```python
from build123d import *

# Parameters (mm, degrees)
SKETCH_1_W          = 40
SKETCH_1_H          = 39
SKETCH_1_R          = 2
EXTRUDE_2_DEPTH     = 20
SKETCH_4_R          = 2
CUT_EXTRUDE_1_DEPTH = 20
SKETCH_5_R          = 4
EXTRUDE_3_DEPTH     = 1
SKETCH_6_R          = 3
EXTRUDE_4_DEPTH     = 0.5
SKETCH_7_R          = 1.5
EXTRUDE_5_DEPTH     = 4.5
FILLET_2_R          = 3
FILLET_3_R          = 3
FILLET_4_R          = 1
FILLET_5_R          = 1
FILLET_6_R          = 1
FILLET_8_R          = 1


with BuildPart() as part:
    # 草图1 → 凸台-拉伸2 (new body)
    with BuildSketch(Plane.XY):
        Rectangle(SKETCH_1_W, SKETCH_1_H)
        with BuildLine():
            Line((-20, 7.5), (-20, 11.5))
            Line((-20, 11.5), (-24, 11.5))
            ThreePointArc((-24, 11.5), (-22.585786438, 10.914213562), (-22, 9.5))
            ThreePointArc((-22, 9.5), (-22.585786438, 8.085786438), (-24, 7.5))
            Line((-24, 7.5), (-20, 7.5))
        make_face()
        with BuildLine():
            ThreePointArc((-24, 7.5), (-26, 9.5), (-24, 11.5))
            Line((-24, 11.5), (-27, 11.5))
            Line((-27, 11.5), (-27, 7.5))
            Line((-27, 7.5), (-24, 7.5))
        make_face()
        with Locations((-24, 9.5)):
            Circle(SKETCH_1_R)
        Polygon((27, 11.5), (20, 11.5), (20, 7.5), (24, 7.5), (27, 7.5), align=None)
    extrude(amount=EXTRUDE_2_DEPTH)

    # 草图4 → 切除-拉伸1 (cut)
    with BuildSketch(Plane(origin=(0, 19.5, 0), x_dir=(1, 0, 0), z_dir=(0, 1, 0))):
        with Locations((-24, -15)):
            Circle(SKETCH_4_R)
        with Locations((24, -15)):
            Circle(SKETCH_4_R)
        with Locations((-24, -5)):
            Circle(SKETCH_4_R)
        with Locations((24, -5)):
            Circle(SKETCH_4_R)
    extrude(amount=-CUT_EXTRUDE_1_DEPTH, mode=Mode.SUBTRACT)

    # 草图5 → 凸台-拉伸3 (add)
    with BuildSketch(Plane(origin=(0, 19.5, 0), x_dir=(1, 0, 0), z_dir=(0, 1, 0))):
        with Locations((-10, -10)):
            Circle(SKETCH_5_R)
    extrude(amount=EXTRUDE_3_DEPTH)

    # 草图6 → 凸台-拉伸4 (add)
    with BuildSketch(Plane(origin=(0, 20.5, 0), x_dir=(1, 0, 0), z_dir=(0, 1, 0))):
        with Locations((-10, -10)):
            Circle(SKETCH_6_R)
    extrude(amount=EXTRUDE_4_DEPTH)

    # 草图7 → 凸台-拉伸5 (add)
    with BuildSketch(Plane(origin=(0, 21, 0), x_dir=(1, 0, 0), z_dir=(0, 1, 0))):
        with Locations((-10, -10)):
            Circle(SKETCH_7_R)
    extrude(amount=EXTRUDE_5_DEPTH)

    # 圆角2
    fillet_2_edges = [part.edges().sort_by_distance(p)[0] for p in [
        (-20, 15.5, 20),
    ]]
    fillet(fillet_2_edges, radius=FILLET_2_R)

    # 圆角3
    fillet_3_edges = [part.edges().sort_by_distance(p)[0] for p in [
        (-20, 15.5, 0),
        (20, 15.5, 0),
        (20, 15.5, 20),
    ]]
    fillet(fillet_3_edges, radius=FILLET_3_R)

    # 圆角4
    fillet_4_edges = [part.edges().sort_by_distance(p)[0] for p in [
        (20, -6, 0),
        (0, -19.5, 0),
        (-20, -6, 0),
        (20, -19.5, 10),
        (-20, -19.5, 10),
        (-20, -6, 20),
        (0, -19.5, 20),
        (20, -6, 20),
    ]]
    fillet(fillet_4_edges, radius=FILLET_4_R)

    # 圆角5
    fillet_5_edges = [part.edges().sort_by_distance(p)[0] for p in [
        (-27, 9.5, 0),
        (-27, 9.5, 20),
    ]]
    fillet(fillet_5_edges, radius=FILLET_5_R)

    # 圆角6
    fillet_6_edges = [part.edges().sort_by_distance(p)[0] for p in [
        (19.121320344, 19.5, 0.878679656),
        (19.121320344, 19.5, 19.121320344),
        (0, 19.5, 20),
        (-20, 19.5, 10),
        (-19.121320344, 19.5, 19.121320344),
        (20, 19.5, 10),
        (0, 19.5, 0),
        (-19.121320344, 19.5, 0.878679656),
    ]]
    fillet(fillet_6_edges, radius=FILLET_6_R)

    # 圆角8
    fillet_8_edges = [part.edges().sort_by_distance(p)[0] for p in [
        (27, 9.5, 0),
        (27, 9.5, 20),
    ]]
    fillet(fillet_8_edges, radius=FILLET_8_R)


solid = part.part
```
Work out the finished part from the listing and answer in its coordinate system (mm). A direction names the side the tool comes from. Round coordinates to 2 decimals unless told otherwise and drop trailing zeros. Loops run counter-clockwise (first coordinate to the right, second up) from the corner with the lowest first, then second, coordinate; pieces in that order, holes last. Notation, with made-up numbers: (47, 56) -> (53, 56) arc R21 cw to (53, 86) -> close; hole circle Ø6 at (15.25, 74.5). An arc over 180 degrees is marked (long way). Write each question's results on one line, items separated by ' | '. Start each with the question number.
1. Section C-C (y = 0) is taken. Determine the outline of the cut face in (x, z).
2. For a pull along Z with two mould halves and no side action, classify faces 5 (the face through (0, -19.5, 10)), 6 (the face through (-25.474, 9.528, 13.648)), 7 (the face through (0, 0, 0)) as +Z half, -Z half, draft (parallel to the pull), parting line (faces both ways), or undercut.
3. Find the intervals of material crossed by probe 1 along X at (y, z) = (9.15, 15); probe 2 along Z at (x, y) = (24, 8.85); probe 3 along X at (y, z) = (8.5, 14), in increasing order. Write a range as from..to.
4. Given pin 1 Ø8 at (x, z) = (-23, 11) entering from +Y; pin 2 Ø2 at (y, z) = (13.5, 7.5) entering from +X; pin 3 Ø5 at (y, z) = (-12.5, 7.5) entering from -X; pin 4 Ø3.5 at (x, z) = (24, 5) entering from +Y, each flat-ended and moving along its own axis, determine where each tip first touches the part or whether it passes through.
5. A tool of negligible diameter and unlimited length cuts with its end or side. For faces 1 (the face through (-20, -6, 10)), 2 (the face through (20, 15, 10)), 3 (the face through (-8.7, 21, 11.3)), 4 (the face through (20, -6, 10)), from which of +Z, -Z, +X, -X, +Y, -Y can it reach the whole face along a straight path? Write none if from no direction.
6. Section A-A (x = 24) is taken. Determine the outline of the cut face in (y, z), plus the area to 3 significant figures.
7. Section B-B (z = 5) is taken. Determine the outline of the cut face in (x, y).
8. Section D-D (x = -10) is taken. Determine the outline of the cut face in (y, z).
Evaluation:
1) outline: (-20, 1) arc R1 ccw to (-19, 0) -> (19, 0) arc R1 ccw to (20, 1) -> (20, 19) arc R1 ccw to (19, 20) -> (-19, 20) arc R1 ccw to (-20, 19) -> close
2) face 5: draft | face 6: undercut | face 7: -Z half
3) probe 1: x = -27..-26, -22..22, 26..27 | probe 2: z = 0..3, 7..13, 17..20 | probe 3: x = -27..-25.73, -22.27..22.27, 25.73..27
4) pin 1: stops at y = 19.5 | pin 2: stops at x = 20 | pin 3: stops at x = -20 | pin 4: passes through
5) face 1: +Z, -Z, -X, -Y | face 2: +Z, -Z, +X, +Y | face 3: +Y | face 4: +Z, -Z, +X, -Y
6) outline: (7.5, 0) -> (11.5, 0) -> (11.5, 3) -> (7.5, 3) -> close; (7.5, 7) -> (11.5, 7) -> (11.5, 13) -> (7.5, 13) -> close; (7.5, 17) -> (11.5, 17) -> (11.5, 20) -> (7.5, 20) -> close | area: 48.0 mm2
7) outline: (-27, 7.5) -> (-26, 7.5) -> (-26, 11.5) -> (-27, 11.5) -> close; (-22, 7.5) -> (-20, 7.5) -> (-20, -18.5) arc R1 ccw to (-19, -19.5) -> (19, -19.5) arc R1 ccw to (20, -18.5) -> (20, 7.5) -> (22, 7.5) -> (22, 11.5) -> (20, 11.5) -> (20, 18.5) arc R1 ccw to (19, 19.5) -> (-19, 19.5) arc R1 ccw to (-20, 18.5) -> (-20, 11.5) -> (-22, 11.5) -> close; (26, 7.5) -> (27, 7.5) -> (27, 11.5) -> (26, 11.5) -> close
8) outline: (-19.5, 1) arc R1 ccw to (-18.5, 0) -> (18.5, 0) arc R1 ccw to (19.5, 1) -> (19.5, 6) -> (20.5, 6) -> (20.5, 7) -> (21, 7) -> (21, 8.5) -> (25.5, 8.5) -> (25.5, 11.5) -> (21, 11.5) -> (21, 13) -> (20.5, 13) -> (20.5, 14) -> (19.5, 14) -> (19.5, 19) arc R1 ccw to (18.5, 20) -> (-18.5, 20) arc R1 ccw to (-19.5, 19) -> close
